Input: part model. Units: mm. Frame: model coordinates. Face numbers are marked on the shaded views. A direction names the side the tool comes from. Give positions to 0.01 mm unless a question says otherwise; leave off trailing zeros. Write each loop counter-clockwise with the first axis right and the second up, starting at its lowest first coordinate (ties: lowest second). Pieces come first, ordered by that corner, then holes. Notation, with made-up numbers: (23, 82.5) - (52, 82.5) arc R7 cw to (52, 92.5) - close; hole circle Ø6 at (-11, -21.5). An arc over 180 degrees is marked (long way). Answer as CSV lines item,"result". Start each with the question number.
from build123d import *

# Parameters (mm, degrees)
HEX_DIE_START = -2e-06
SKETCH2_R     = 10.00506
HEX_DIE_DEPTH = 7.493002
SKETCH3_W     = 16.483602772
SKETCH3_H     = 2.3876
SLOT_DEPTH    = 4.2672
SKETCH4_R     = 6.245225
INDENT_DEPTH  = 0.936625


with BuildPart() as part:
    # BodySke → Base-Revolve (revolve)
    with BuildSketch(Plane.XY, mode=Mode.PRIVATE) as base_revolve_sk:
        Polygon((9.0932, 4.7625), (9.0932, 9.906), (7.493, 9.906), (7.493, 8.241801386), (0.637626437, 8.241801386), (0, 7.1374), (0, 0), (44.0182, 0), (44.0182, 4.7625), align=None)
    revolve(base_revolve_sk.sketch.rotate(Axis((-25.4, 0, 0), (1, 0, 0)), 90), axis=Axis((-25.4, 0, 0), (1, 0, 0)))

    # Sketch2 → Hex-Die (cut)
    with BuildSketch(Plane(origin=(0, 0, 0), x_dir=(0, 0, -1), z_dir=(1, 0, 0)).offset(HEX_DIE_START)):
        Circle(SKETCH2_R)
        Polygon((-7.1374, 4.120779829), (0, 8.241559659), (7.1374, 4.120779829), (7.1374, -4.120779829), (0, -8.241559659), (-7.1374, -4.120779829), align=None, mode=Mode.SUBTRACT)
    extrude(amount=HEX_DIE_DEPTH, mode=Mode.SUBTRACT)

    # Sketch3 → Slot (cut)
    with BuildSketch(Plane(origin=(0, 0, 0), x_dir=(0, 0, -1), z_dir=(1, 0, 0))):
        Rectangle(SKETCH3_W, SKETCH3_H)
    extrude(amount=SLOT_DEPTH, mode=Mode.SUBTRACT)

    # Sketch4 → Indent (cut)
    with BuildSketch(Plane(origin=(0, 0, 0), x_dir=(0, 0, -1), z_dir=(1, 0, 0))):
        Circle(SKETCH4_R)
    extrude(amount=INDENT_DEPTH, mode=Mode.SUBTRACT)


solid = part.part
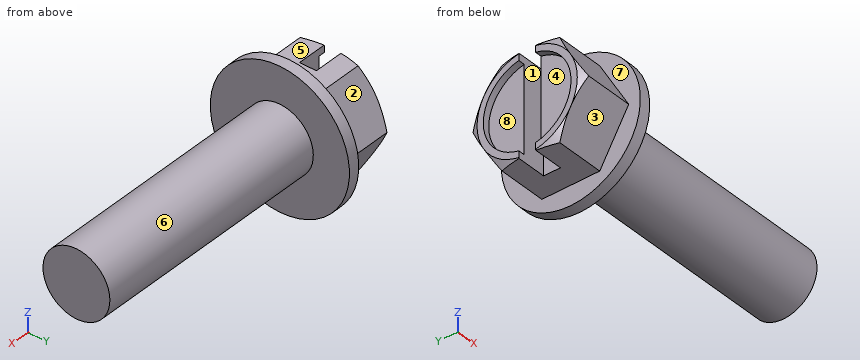
1) Cut plane B-B on x = 29. Output: boundary loops of the cut face in (y, z) (1 decimal), and give its area (3 significant figures).
2) Contact query for flat-ended pins moving along their axis: P1, Ø5.5, axis at y = -4, z = -2.5, coming from the -X side; P2, Ø6, axis at y = 2, z = 1, coming from the -X side; P3, Ø2, axis at x = 9, z = 8, coming from the -Y side; P4, Ø3.5, axis at x = 4.5, y = -1.5, coming from the +Z side. Output: stop coordinate, or through.
3) Reachability of the marked faces 1, 2, 3, 4 and 5 from +Z, -Z, +X, -X, +Y, -Y: full face, straight path, thin tool, end or side. Return the list, or none.
4) Material intervals for line 1 (Y direction, x = 19, z = 0); line 2 (X direction, y = -7, z = 3.25); line 3 (X direction, y = -2.25, z = -2.5), sorted ascending. Write a range as from..to.
5) Cut plane A-A on y = 0. Output: boundary loops of the cut face in (x, z), and give its area (3 significant figures).
6) Pull-direction query (Y, two-part tool) for the marked faces 6, 7 and 8; classes: +Y half, -Y half, draft (parallel to the pull), parting line (faces both ways), or undercut.
Numbers:
1,outline,"circle Ø9.5 at (0, 0)"
1,area,"71.3 mm²"
2,P1,"stops at x = 0"
2,P2,"stops at x = 0.94"
2,P3,"stops at y = -7.01"
2,P4,"stops at z = 7.14"
3,face 1,"+Z, -Z, -X"
3,face 2,"+Z, -X, +Y"
3,face 3,"-Z, -X, -Y"
3,face 4,"-X"
3,face 5,"+Z, -X, +Y, -Y"
4,line 1,"y = -4.76..4.76"
4,line 2,"x = 7.49..9.09"
4,line 3,"x = 0.94..44.02"
5,outline,"(4.27, -7.14) - (7.49, -7.14) - (7.49, -9.91) - (9.09, -9.91) - (9.09, -4.76) - (44.02, -4.76) - (44.02, 4.76) - (9.09, 4.76) - (9.09, 9.91) - (7.49, 9.91) - (7.49, 7.14) - (4.27, 7.14) - close"
5,area,"410 mm²"
6,face 6,"parting line"
6,face 7,"draft"
6,face 8,"undercut"
